Can you work these out from the model? Positions are in its coordinate system, mm. A direction names the side the tool comes from. Give positions to 0.01 mm unless a question says otherwise; leave off trailing zeros. Write each loop counter-clockwise with the first axis right and the second up, starting at its lowest first coordinate (ties: lowest second). Pieces come first, ordered by that corner, then holes. Notation, with made-up numbers: (-34, 14.5) - (-1, 14.5) arc R28 ccw to (-1, 36.5) - close; hole circle Ø2 at (56, 52). An arc over 180 degrees is marked (long way). Use a Markdown table: item, result. Add a question column.
```python
from build123d import *

# Parameters (mm, degrees)
SKETCH3_R           = 3.96875
SKETCH3_R_2         = 3.175
BOSS_EXTRUDE1_DEPTH = 6.35
SKETCH4_W           = 1.27
SKETCH4_H           = 1.27


with BuildPart() as part:
    # Sketch3 → Boss-Extrude1 (new body)
    with BuildSketch(Plane.XY):
        with BuildLine():
            Line((7.14375, 19.05), (7.14375, 0))
            ThreePointArc((7.14375, 0), (0, -7.14375), (-7.14375, 0))
            Line((-7.14375, 0), (-7.14375, 19.05))
            Line((-7.14375, 19.05), (-24.65552597, 33.744124757))
            Line((-24.65552597, 33.744124757), (-49.669642896, 38.15478847))
            ThreePointArc((-49.669642896, 38.15478847), (-53.394417896, 43.474318461), (-48.074887905, 47.199093461))
            Line((-48.074887905, 47.199093461), (-20.63735676, 42.361116436))
            Line((-20.63735676, 42.361116436), (7.14375, 19.05))
        make_face()
        Circle(SKETCH3_R, mode=Mode.SUBTRACT)
        with Locations((0, 12.7)):
            Circle(SKETCH3_R_2, mode=Mode.SUBTRACT)
    extrude(amount=BOSS_EXTRUDE1_DEPTH)

    # Cut-Sweep1: sweep along a path in Sketch6
    with BuildLine(Plane(origin=(0, 0, 0), x_dir=(-1, 0, 0), z_dir=(0, 0, -1))) as cut_sweep1_path:
        Line((48.074887905, 47.199093461), (20.63735676, 42.361116436))
        Line((20.63735676, 42.361116436), (-7.14375, 19.05))
        Line((-7.14375, 19.05), (-7.14375, 0))
        ThreePointArc((-7.14375, 0), (0, -7.14375), (7.14375, 0))
    # Sketch4 → Cut-Sweep1 (sweep, cut)
    with BuildSketch(Plane(origin=(-48.074887905, 0, 0), x_dir=(0, 0, -1), z_dir=(1, 0, 0))):
        with Locations((-3.175, 46.564093461)):
            Rectangle(SKETCH4_W, SKETCH4_H)
    sweep(path=cut_sweep1_path.line, transition=Transition.RIGHT, mode=Mode.SUBTRACT)


solid = part.part
```
Q1. Suppose I cut it at B-B (y = 12.7). Please give me the cut outline in (x, z) (3 decimals), and give its area (3 significant figures).
Q2. I'm going to push flat-ended pins straight in: P1, Ø5, axis at x = -21.5, y = 26.5, coming from the +Z side; P2, Ø1.4, axis at y = 7.5, z = 3, coming from the +X side; P3, Ø1.9, axis at y = 5, z = 3.5, coming from the -X side; P4, Ø2, axis at x = -23.5, z = 3, coming from the +Y side. Where does each tip first touch, or does it pass through?
Q3. On a 3-axis mill with a long thin cutter (end or side, diameter ignored), from which of +Z, -Z, +X, -X, +Y, -Y can I reach the whole of each face in a straight line? I mean faces 1 (the flat face through (-34.441, 43.525, 3.184)), 2 (the flat face through (-36.99, 35.92, 3.13)), 3 (the flat face through (5.893, 9, 3)). Say none if no direction works.
Q4. Suppose I cut it at C-C (x = 0). Please give me the cut outline in (y, z) (3 decimals).
Q5. If I drill on probe 1 along Y at (x, z) = (0, 3.75) (3 decimals); probe 2 along Z at (x, y) = (-28.5, 43); probe 3 along Y at (x, z) = (2.5, 1), over which ranges is the centre line in solid material (lowest first)? Write a range as [from, to].
Q6. Suppose I cut it at A-A (z = 1.5). Give the number of separate pieces and of enclosed holes in the cut face, and give its area (3 significant figures).
Q7. Suppose I cut it at D-D (x = -38). Please give me the cut outline in (y, z).
Q8. If we mould it in two halves opening along X, with no side actions, what happens to faces 4 (the cylindrical face through (0.16, -7.14, 5.06)), 5 (the flat face through (7.144, 10, 5)), 6 (the cylindrical face through (1.5, 9.9, 3.1)), 7 (the flat face through (-15.777, 26.294, 3.131))? For each: released by +X, released by -X, zero draft, split by the parting line, or undercut.
Derived:
| question | item | result |
|---|---|---|
| 1 | outline | (-7.144, 0) - (-3.175, 0) - (-3.175, 6.35) - (-7.144, 6.35) - close; (3.175, 0) - (7.144, 0) - (7.144, 2.54) - (5.893, 2.54) - (5.893, 3.81) - (7.144, 3.81) - (7.144, 6.35) - (3.175, 6.35) - close |
| 1 | area | 48.8 mm² |
| 2 | P1 | through |
| 2 | P2 | x = 7.14 |
| 2 | P3 | x = -7.14 |
| 2 | P4 | y = 43.02 |
| 3 | face 1 | +X, +Y |
| 3 | face 2 | +Z, -Z, -X, -Y |
| 3 | face 3 | +X, +Y, -Y |
| 4 | outline | (-7.144, 0) - (-3.969, 0) - (-3.969, 6.35) - (-7.144, 6.35) - (-7.144, 3.81) - (-5.897, 3.81) - (-5.897, 2.54) - (-7.144, 2.54) - close; (3.969, 0) - (9.525, 0) - (9.525, 6.35) - (3.969, 6.35) - close; (15.875, 0) - (25.044, 0) - (25.044, 2.54) - (23.412, 2.54) - (23.412, 3.81) - (25.044, 3.81) - (25.044, 6.35) - (15.875, 6.35) - close |
| 5 | probe 1 | [-5.897, -3.969], [3.969, 9.525], [15.875, 23.412] |
| 5 | probe 2 | [0, 2.54], [3.81, 6.35] |
| 5 | probe 3 | [-6.69, -3.08], [3.08, 10.74], [14.66, 22.95] |
| 6 | separate pieces | 1 |
| 6 | enclosed holes | 2 |
| 6 | area | 820 mm² |
| 7 | outline | (36.1, 0) - (45.42, 0) - (45.42, 2.54) - (44.15, 2.54) - (44.15, 3.81) - (45.42, 3.81) - (45.42, 6.35) - (36.1, 6.35) - close |
| 8 | face 4 | split by the parting line |
| 8 | face 5 | released by +X |
| 8 | face 6 | undercut |
| 8 | face 7 | released by -X |
